Could you check a few things on this model? Use its own coordinates, in mm. Give positions to 0.01 mm unless a question says otherwise; leave off trailing zeros. Order: outer loops, then holes, each group sorted by start corner. A loop starts at its lowest first (then second) coordinate and runs counter-clockwise, first axis right, second up. Notation, with made-up numbers: M 81,-6.75 L 123,-6.75 A28 ccw 123,11.25 Z; hole C -21,24.25 d2. An arc over 180 degrees is marked long. Use a Markdown table: item, result. Add a question column.
Item 1: If I drill on L1, parallel to Y at x = 27, z = 0.5; L2, parallel to X at y = 3, z = 0.7; L3, parallel to X at y = -3.75, z = 0.9, over which ranges is the centre line in solid material (lowest first)? Write a range as from..to.
Item 2: Suppose I cut it at D-D on y = -2.75. Write out the boundary of the cut face in (x, z), plus the area to 3 significant figures.
Item 3: Suppose I cut it at C-C on y = -5.5. Write out the boundary of the cut face in (x, z).
Item 4: Suppose I cut it at A-A on z = 0.15. Count the separate pieces of the cut face and the enclosed holes in it, plus the area to 3 significant figures.
Item 5: Suppose I cut it at B-B on x = 0. Write out the boundary of the cut face in (y, z).
Item 6: I'm going to push flat-ended pins straight in: pin 1 Ø0.5 at (x, z) = (26, 0.5) entering from -Y; pin 2 Ø1.4 at (x, y) = (24.75, 0) entering from -Z; pin 3 Ø5 at (x, y) = (1.5, -6.5) entering from +Z. Where does each tip first touch, or does it pass through?
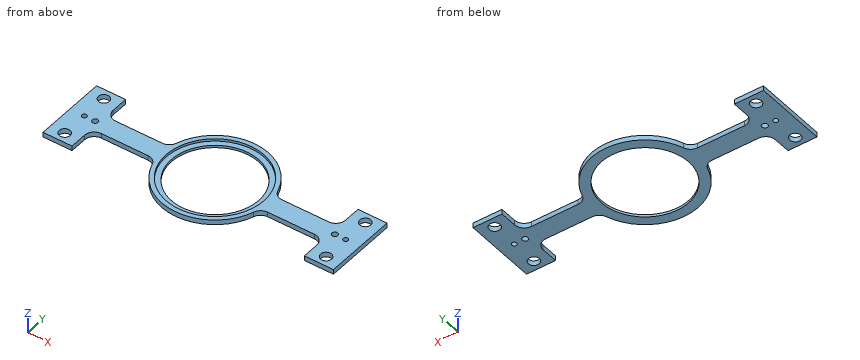
from build123d import *

# Parameters (mm, degrees)
SKETCH1_R             = 9
BOSS_EXTRUDE1_DEPTH   = 1
SKETCH2_R             = 10.1
CUT_EXTRUDE1_DEPTH    = 0.5
SKETCH6_R             = 0.5
CUT_EXTRUDE3_DEPTH    = 32.968734726
F_1_CLEARANCE_HOLE1_D = 2.2606
F_0_80_TAPPED_HOLE1_D = 1.19126
FILLET1_R             = 2


with BuildPart() as part:
    # Sketch1 → Boss-Extrude1 (new body)
    with BuildSketch(Plane.XY):
        with BuildLine():
            Line((10.816653826, 2), (24, 2))
            Line((24, 2), (24, 7.5))
            Line((24, 7.5), (30, 7.5))
            Line((30, 7.5), (30, -7.5))
            Line((30, -7.5), (24, -7.5))
            Line((24, -7.5), (24, -2))
            Line((24, -2), (10.816653826, -2))
            ThreePointArc((10.816653826, -2), (0, -11), (-10.816653826, -2))
            Line((-10.816653826, -2), (-24, -2))
            Line((-24, -2), (-24, -7.5))
            Line((-24, -7.5), (-30, -7.5))
            Line((-30, -7.5), (-30, 7.5))
            Line((-30, 7.5), (-24, 7.5))
            Line((-24, 7.5), (-24, 2))
            Line((-24, 2), (-10.816653826, 2))
            ThreePointArc((-10.816653826, 2), (0, 11), (10.816653826, 2))
        make_face()
        Circle(SKETCH1_R, mode=Mode.SUBTRACT)
    extrude(amount=BOSS_EXTRUDE1_DEPTH)

    # Sketch2 → Cut-Extrude1 (cut)
    with BuildSketch(Plane.XY.offset(1)):
        Circle(SKETCH2_R)
    extrude(amount=-CUT_EXTRUDE1_DEPTH, mode=Mode.SUBTRACT)

    # Sketch6 → Cut-Extrude3 (cut, through all)
    with BuildSketch(Plane(origin=(0, 0, 0), x_dir=(-1, 0, 0), z_dir=(0, 0, -1))):
        with Locations((-27, 0)):
            Circle(SKETCH6_R)
        with Locations((27, 0)):
            Circle(SKETCH6_R)
    extrude(amount=-CUT_EXTRUDE3_DEPTH, mode=Mode.SUBTRACT)

    # #1 Clearance Hole1 (through all)
    with Locations(Plane(origin=(0, 0, 0), x_dir=(-1, 0, 0), z_dir=(0, 0, -1))):
        with Locations((-27, -5.5), (-27, 5.5), (27, 5.5), (27, -5.5)):
            Hole(F_1_CLEARANCE_HOLE1_D / 2)

    # #0-80 Tapped Hole1 (through all)
    with Locations(Plane(origin=(0, 0, 0), x_dir=(-1, 0, 0), z_dir=(0, 0, -1))):
        with Locations((-24.75, 0), (24.75, 0)):
            Hole(F_0_80_TAPPED_HOLE1_D / 2)

    # Fillet1
    fillet1_edges = [part.edges().sort_by_distance(p)[0] for p in [
        (-24, 2, 0.5),
        (-10.816653826, 2, 0.5),
        (10.816653826, 2, 0.5),
        (24, 2, 0.5),
        (24, -2, 0.5),
        (10.816653826, -2, 0.5),
        (-10.816653826, -2, 0.5),
        (-24, -2, 0.5),
    ]]
    fillet(fillet1_edges, radius=FILLET1_R)


solid = part.part
Findings below:
| question | item | result |
|---|---|---|
| 1 | L1 | y = -7.5..-6.63, -4.37..-0.5, 0.5..4.37, 6.63..7.5 |
| 1 | L2 | x = -30..-23.73, -10.64..-9.64, 9.64..10.64, 23.73..30 |
| 1 | L3 | x = -30..-23.98, -10.34..-9.38, 9.38..10.34, 23.98..30 |
| 2 | outline | M -30,0 L -23.56,0 L -23.56,1 L -30,1 Z; M -10.81,0 L -8.57,0 L -8.57,0.5 L -9.72,0.5 L -9.72,1 L -10.81,1 Z; M 8.57,0 L 10.81,0 L 10.81,1 L 9.72,1 L 9.72,0.5 L 8.57,0.5 Z; M 23.56,0 L 30,0 L 30,1 L 23.56,1 Z |
| 2 | area | 16.2 mm^2 |
| 3 | outline | M -30,0 L -28.13,0 L -28.13,1 L -30,1 Z; M -25.87,0 L -24,0 L -24,1 L -25.87,1 Z; M -9.53,0 L -7.12,0 L -7.12,0.5 L -8.47,0.5 L -8.47,1 L -9.53,1 Z; M 7.12,0 L 9.53,0 L 9.53,1 L 8.47,1 L 8.47,0.5 L 7.12,0.5 Z; M 24,0 L 25.87,0 L 25.87,1 L 24,1 Z; M 28.13,0 L 30,0 L 30,1 L 28.13,1 Z |
| 4 | separate pieces | 1 |
| 4 | enclosed holes | 9 |
| 4 | area | 395 mm^2 |
| 5 | outline | M -11,0 L -9,0 L -9,0.5 L -10.1,0.5 L -10.1,1 L -11,1 Z; M 9,0 L 11,0 L 11,1 L 10.1,1 L 10.1,0.5 L 9,0.5 Z |
| 6 | pin 1 | stops at y = -7.5 |
| 6 | pin 2 | stops at z = 0 |
| 6 | pin 3 | stops at z = 0.5 |
